Here's how the part is built. I have some questions about the finished solid (model axes, mm). Coordinates: 2 decimals unless noted, no trailing zeros. Write each loop counter-clockwise with the first axis right and the second up, starting at its lowest first coordinate (ties: lowest second). Pieces come first, ordered by that corner, then holes.
Item 1: I want a section at A-A (y = 141). Please give me the cut outline in (x, z).
Item 2: Please list where these lines run through material, in increasing order: line 1 (Z direction, x = -33.75, y = 107.5); line 2 (Z direction, x = -32.75, y = 220); line 3 (Y direction, x = -30, z = -61).
Item 3: I'm going to push flat-ended pins straight in: P1, Ø3, axis at x = -30.5, z = -52, coming from the -Y side; P2, Ø1.9, axis at x = -32.5, y = 91, coming from the +Z side; P3, Ø1.9, axis at x = -33, y = 93.5, coming from the -Z side. Where does each tip first touch, or does it pass through?
Item 4: I want a section at B-B (z = -124.5). Please give me the cut outline in (x, y), and give its area (3 significant figures).
from build123d import *

# Parameters (mm, degrees)
BOSS_EXTRUDE1_DEPTH = 3.175
CUT_EXTRUDE1_DEPTH  = 6.35
SKETCH3_W           = 6.35
SKETCH3_H           = 25.4
BOSS_EXTRUDE2_DEPTH = 6.35
LPATTERN1_COUNT     = 5
LPATTERN1_PITCH     = 38.1
SKETCH4_W           = 6.35
SKETCH4_H           = 25.4
BOSS_EXTRUDE3_DEPTH = 6.35
LPATTERN2_COUNT     = 3
LPATTERN2_PITCH     = 50.8
CUT_EXTRUDE2_DEPTH  = 6.35
CUT_EXTRUDE3_DEPTH  = 6.35


with BuildPart() as part:
    # Sketch1 → Boss-Extrude1 (new, symmetric)
    with BuildSketch(Plane.ZY.offset(32.038437852)):
        Polygon((-215.9, 95.25), (-215.9, 174.9125), (-29.333338138, 282.626812448), (-29.333338138, 95.25), align=None)
    extrude(amount=BOSS_EXTRUDE1_DEPTH, both=True)

    # Sketch2 → Cut-Extrude1 (cut)
    with BuildSketch(Plane.ZY.offset(35.213437852)):
        Polygon((-190.5, 160.247803163), (-190.5, 120.65), (-54.733338138, 120.65), (-54.733338138, 238.632721936), align=None)
    extrude(amount=-CUT_EXTRUDE1_DEPTH, mode=Mode.SUBTRACT)

    # Sketch3 → Boss-Extrude2 (add)
    with BuildSketch(Plane(origin=(0, 224.671817339, -129.71433422), x_dir=(1, 0, 0), z_dir=(0, 0.8660254037844386, -0.5000000000000001))):
        with Locations((-32.038437852, 61.418634677)):
            Rectangle(SKETCH3_W, SKETCH3_H)
    boss_extrude2 = extrude(amount=BOSS_EXTRUDE2_DEPTH)

    # LPattern1: Boss-Extrude2 ×5
    with Locations(*[Vector(1.0927391974657063e-15, 0.5000000000000003, 0.8660254037844386) * (i * LPATTERN1_PITCH) for i in range(1, LPATTERN1_COUNT)]):
        add(boss_extrude2)

    # Sketch4 → Boss-Extrude3 (add)
    with BuildSketch(Plane.XZ.offset(-95.25)):
        with Locations((-32.038437852, -67.433338138)):
            Rectangle(SKETCH4_W, SKETCH4_H)
    boss_extrude3 = extrude(amount=BOSS_EXTRUDE3_DEPTH)

    # LPattern2: Boss-Extrude3 ×3
    with Locations(*[(0, 0, -i * LPATTERN2_PITCH) for i in range(1, LPATTERN2_COUNT)]):
        add(boss_extrude3)

    # Sketch5 → Cut-Extrude2 (cut)
    with BuildSketch(Plane(origin=(-28.863437852, 0, 0), x_dir=(0, 0, -1), z_dir=(1, 0, 0))):
        Polygon((196.683069069, 95.25), (200.950269069, 95.25), (200.950269069, 104.013), (203.261669069, 104.013), (203.261669069, 107.188), (200.950269069, 107.188), (200.950269069, 110.49), (196.683069069, 110.49), (196.683069069, 107.188), (194.371669069, 107.188), (194.371669069, 104.013), (196.683069069, 104.013), align=None)
        Polygon((39.899738138, 95.25), (44.166938138, 95.25), (44.166938138, 104.013), (46.478338138, 104.013), (46.478338138, 107.188), (44.166938138, 107.188), (44.166938138, 110.49), (39.899738138, 110.49), (39.899738138, 107.188), (37.588338138, 107.188), (37.588338138, 104.013), (39.899738138, 104.013), align=None)
    extrude(amount=-CUT_EXTRUDE2_DEPTH, mode=Mode.SUBTRACT)

    # Sketch6 → Cut-Extrude3 (cut)
    with BuildSketch(Plane(origin=(-28.863437852, 0, 0), x_dir=(0, 0, -1), z_dir=(1, 0, 0))):
        Polygon((206.749229173, 180.1957), (203.05372557, 182.3293), (198.67222557, 174.740319387), (196.670494452, 175.896019387), (195.082994452, 173.14638873), (197.08472557, 171.99068873), (195.43372557, 169.131072846), (199.129229173, 166.997472846), (200.780229173, 169.85708873), (202.781960292, 168.70138873), (204.369460292, 171.451019387), (202.367729173, 172.606719387), align=None)
        Polygon((69.267696323, 259.5707), (65.57219272, 261.7043), (61.19069272, 254.115319387), (59.188961601, 255.271019387), (57.601461601, 252.52138873), (59.60319272, 251.36568873), (57.95219272, 248.506072846), (61.647696323, 246.372472846), (63.298696323, 249.23208873), (65.300427441, 248.07638873), (66.887927441, 250.826019387), (64.886196323, 251.981719387), align=None)
    extrude(amount=-CUT_EXTRUDE3_DEPTH, mode=Mode.SUBTRACT)


solid = part.part
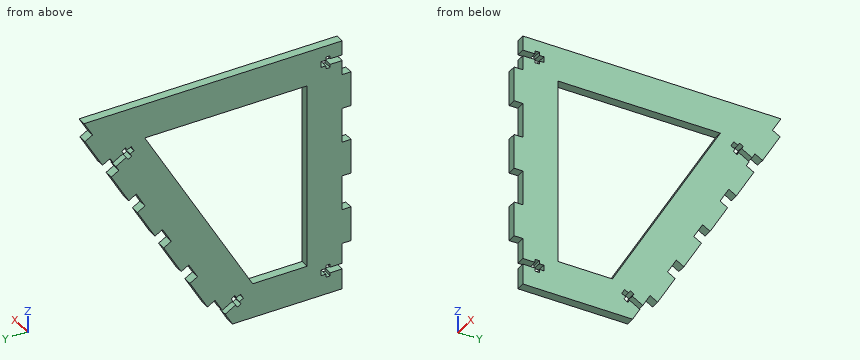
Answer:
1. outline: (-35.21, -215.9) - (-28.86, -215.9) - (-28.86, -190.5) - (-35.21, -190.5) - close; (-35.21, -54.73) - (-28.86, -54.73) - (-28.86, -29.33) - (-35.21, -29.33) - close
2. line 1: z = -215.9 to -200.95, -196.68 to -44.17, -39.9 to -29.33
2. line 2: z = -150.51 to -139.28, -137.81 to -87.01, -54.73 to -29.33
2. line 3: y = 88.9 to 120.65, 235.01 to 246.75, 254.23 to 271.68
3. P1: stops at y = 95.25
3. P2: stops at z = -54.73
3. P3: stops at z = -181.73
4. outline: (-35.21, 88.9) - (-28.86, 88.9) - (-28.86, 120.65) - (-35.21, 120.65) - close; (-35.21, 198.35) - (-28.86, 198.35) - (-28.86, 235.01) - (-35.21, 235.01) - close
4. area: 434 mm2
